Input: part model. Units: mm. Frame: model coordinates. Face numbers are marked on the shaded views. A direction names the side the tool comes from. Coordinates: 2 decimals unless noted, no trailing zeros. Loops run counter-clockwise (first coordinate to the right, second up) from the corner with the lowest first, then second, coordinate; pieces in that order, holes last.
Item 1: Pull-direction query (X, two-part tool) for the marked faces 1, 2, 3 and 4; classes: released by +X, released by -X, zero draft, split by the parting line, or undercut.
Item 2: Contact query for flat-ended pins moving along their axis: P1, Ø1.5, axis at y = 59, z = 1.5, coming from the +X side; P2, Ø2, axis at y = 22.5, z = 2.5, coming from the -X side; P3, Ø2, axis at x = -45.5, y = 65.5, coming from the -Z side. Output: stop coordinate, or through.
Item 3: Section A-A on y = 27. Return loops of the section in (x, z).
Item 4: Section B-B on x = -39.5. Return loops of the section in (y, z), and give its area (3 significant figures).
Item 5: Section D-D on x = -15. Return loops of the section in (y, z).
Item 6: Reachability of the marked faces 5, 6, 7 and 8 from +Z, -Z, +X, -X, +Y, -Y: full face, straight path, thin tool, end or side. Return the list, or none.
Item 7: Ray query, line 1 along X through (y, z) = (39.5, 1.25); line 2 along Z through (x, y) = (-38, 7); line 3 along X through (y, z) = (29, 6.5). Return the intervals inside material, ascending.
```python
from build123d import *

# Parameters (mm, degrees)
F1_DEPTH = 6.5933763981
F3_D     = 19.05
F5_DEPTH = 5.4949615151


with BuildPart() as f1:
    # F0 (on Top) → F1 (new body)
    with BuildSketch(Plane.XY):
        Polygon((-64.5944178104, 68.5121715069), (-64.5944178104, 0), (0, 34.2560857534), align=None)
    extrude(amount=F1_DEPTH)

    # F3 (through all)
    with Locations(Plane.XY.offset(6.5933763981)):
        with Locations((-41.6155830026, 34.2560857534)):
            Hole(F3_D / 2)

    # F4 (on face) → F5 (join)
    with BuildSketch(Plane.XY.offset(6.5933763981)):
        Polygon((-97.2867310047, 34.2560857534), (-64.5944178104, 14.6030057222), (-64.5944178104, 34.2560857534), (-64.5944178104, 53.6291189492), align=None)
        Polygon((-32.2972089052, 17.1280428767), (-53.0271635681, 6.1344132618), (-17.9972769314, -9.8363857863), align=None)
        Polygon((-10.2336501417, 28.8289171419), (-32.2972089052, 17.1280428767), (-17.9972769314, -9.8363857863), align=None)
        Polygon((-20.6264760453, 79.3094929525), (-51.0069840933, 61.306404966), (-32.2972089052, 51.3841286302), (-13.4495195214, 41.3887128393), align=None)
    extrude(amount=-F5_DEPTH)


solid = f1.part
```
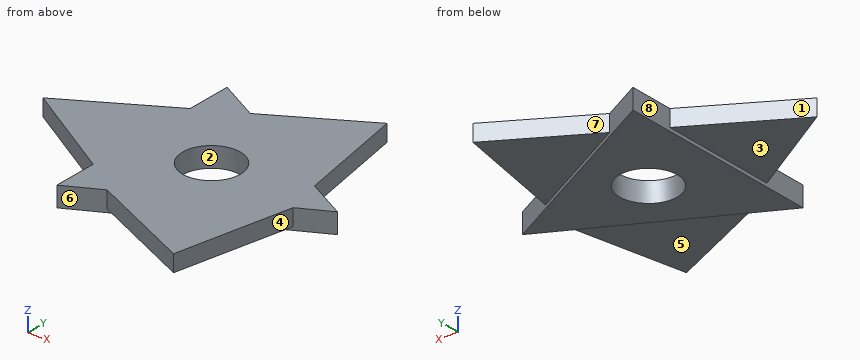
Results found:
1. face 1: released by -X
1. face 2: undercut
1. face 3: zero draft
1. face 4: released by +X
2. P1: stops at x = -16.64
2. P2: stops at x = -79.39
2. P3: stops at z = 1.1
3. outline: (-85.22, 1.1) - (-64.59, 1.1) - (-64.59, 0) - (-47.79, 0) - (-47.79, 6.59) - (-85.22, 6.59) - close; (-35.45, 0) - (-13.68, 0) - (-13.68, 1.1) - (-10.6, 1.1) - (-10.6, 6.59) - (-35.45, 6.59) - close
4. outline: (-0.03, 1.1) - (13.31, 1.1) - (13.31, 0) - (24.97, 0) - (24.97, 6.59) - (-0.03, 6.59) - close; (43.54, 0) - (55.2, 0) - (55.2, 1.1) - (68.13, 1.1) - (68.13, 6.59) - (43.54, 6.59) - close
4. area: 298 mm2
5. outline: (5.09, 1.1) - (26.3, 1.1) - (26.3, 0) - (42.21, 0) - (42.21, 1.1) - (49.58, 1.1) - (49.58, 6.59) - (5.09, 6.59) - close
6. face 5: -Z, +X, -Y
6. face 6: -Z, -Y
6. face 7: +Z, -Z, +Y
6. face 8: -Z, -X
7. line 1: x = -88.44 to -49.57, -33.66 to -9.89
7. line 2: z = 1.1 to 6.59
7. line 3: x = -88.54 to -49.56, -33.67 to -9.91
